The drawing under review shows one solid part. Ordinate dimensions are in mm from its lowest x, y, z. A direction names the side the tool comes from. Coordinates: 2 decimals unless noted, no trailing zeros. Loops run counter-clockwise (first coordinate to the right, second up) from the corner with the lowest first, then second, coordinate; pieces in that order, holes last.
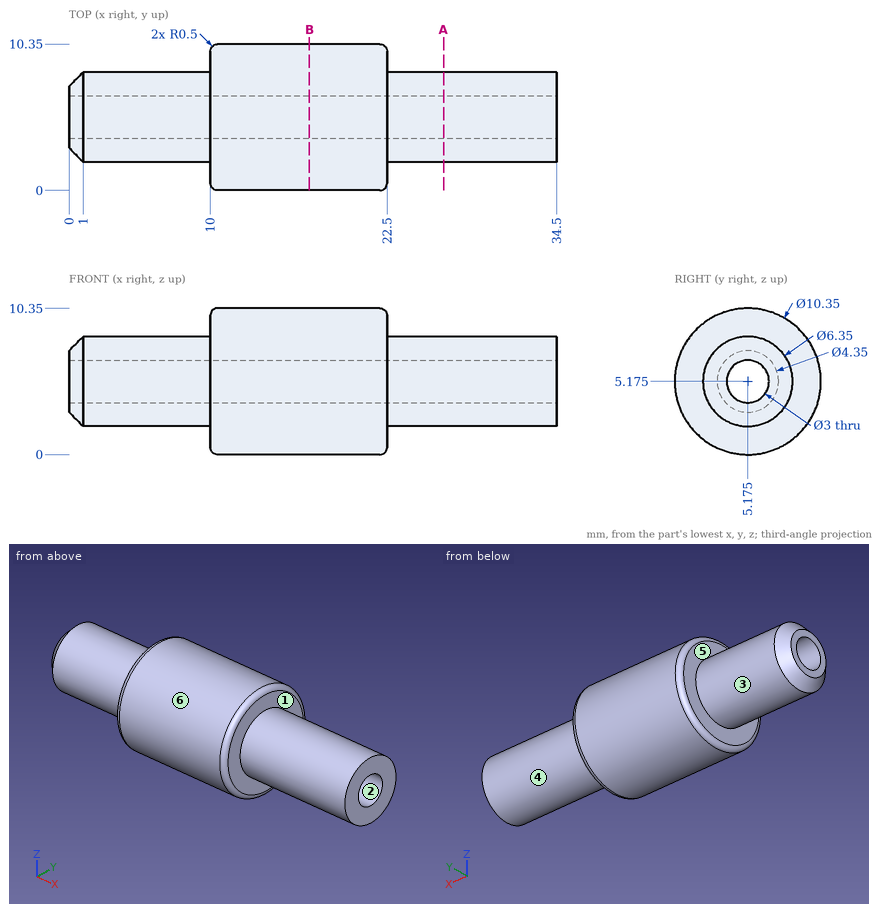
Q1. For line 1 (X direction, y = 8.5, z = 2.25); line 2 (X direction, y = 7.25, z = 4.5); line 3 (Y direction, x = 32.5, z = 4), list the stretches that pass through material, from the lowest coordinate up.
Q2. Clearance check with flat-ended pins moving along their axes: pin 1 Ø4.5 at (y, z) = (5.5, 5) entering from +X; pin 2 Ø4 at (x, z) = (28.5, 1.5) entering from -Y; pin 3 Ø1 at (x, z) = (18.5, 3) entering from -Y; pin 4 Ø1 at (x, z) = (4.5, 4) entering from -Y. State where each tip first meets the part, or that it passes through.
Q3. The part is to be moulded in two halves that separate along Z. For the marked faces 1, 2 and 3, say which applies: pulls with the +Z half, pulls with the -Z half, needs draft (parallel to the pull), parting line crosses it, or undercut.
Q4. Take a section at B-B, the plane x = 17. Write out the cut boundary in (y, z) (3 decimals), then the cut area to 3 significant figures.
Q5. Take a section at A-A, the plane x = 26.5. Write out the cut boundary in (y, z) (3 decimals).
Q6. Machinability: for the marked faces 4, 5 and 6, which of the approach directions +Z, -Z, +X, -X, +Y, -Y give a long, thin tool a straight path to every point of the face, cutting with its end or side? Answer none if there is none.
Entries:
1. line 1: x = 10 to 22.5
1. line 2: x = 0.01 to 34.5
1. line 3: y = 2.23 to 4.24, 6.11 to 8.12
2. pin 1: stops at x = 34.5
2. pin 2: stops at y = 2.48
2. pin 3: stops at y = 0.28
2. pin 4: stops at y = 2.07
3. face 1: needs draft
3. face 2: undercut
3. face 3: parting line crosses it
4. outline: circle Ø10.35 at (5.175, 5.175); hole circle Ø3 at (5.175, 5.175)
4. area: 77.1 mm2
5. outline: circle Ø6.35 at (5.175, 5.175); hole circle Ø3 at (5.175, 5.175)
6. face 4: +X
6. face 5: -X
6. face 6: +X, -X
